Design review of the part built by this model. Coordinates are the model's own, in mm. A direction names the side the tool comes from. Give positions to 0.01 mm unless a question says otherwise; leave off trailing zeros. Order: outer loops, then holes, each group sorted by start corner. A loop starts at its lowest first (then second) coordinate and runs counter-clockwise, first axis right, second up. Notation, with made-up numbers: M -9.75,21 L 43.25,21 A21 cw 43.25,32 Z; hole C 57,86.5 d4. An arc over 180 degrees is marked long. Put each result on its own line as item: value. Start each with the question number.
from build123d import *

# Parameters (mm, degrees)
F0_R     = 1.75
F0_R_2   = 14
F1_DEPTH = 1
F2_W     = 21
F2_H     = 24
F3_DEPTH = 1.001
F4_R     = 2


with BuildPart() as f1:
    # F0 (on Top) → F1 (new body)
    with BuildSketch(Plane.XY):
        Polygon((15.3431457505, 21), (-15.3431457505, 21), (-21, 15.3431457505), (-21, -15.3431457505), (-15.3431457505, -21), (15.3431457505, -21), (21, -15.3431457505), (21, 15.3431457505), align=None)
        with Locations((-15.5, -15.5)):
            Circle(F0_R, mode=Mode.SUBTRACT)
        with Locations((15.5, -15.5)):
            Circle(F0_R, mode=Mode.SUBTRACT)
        with Locations((-15.5, 15.5)):
            Circle(F0_R, mode=Mode.SUBTRACT)
        Circle(F0_R_2, mode=Mode.SUBTRACT)
        with Locations((15.5, 15.5)):
            Circle(F0_R, mode=Mode.SUBTRACT)
    extrude(amount=F1_DEPTH)

    # F2 (on face) → F3 (cut, through all)
    with BuildSketch(Plane.XY.offset(1)):
        with Locations((10.5, 0)):
            Rectangle(F2_W, F2_H)
    extrude(amount=-F3_DEPTH, mode=Mode.SUBTRACT)

    # F4
    f4_edges = [f1.edges().sort_by_distance(p)[0] for p in [
        (7.211103, 12, 0.5),
        (21, 12, 0.5),
        (21, -12, 0.5),
        (7.211103, -12, 0.5),
    ]]
    fillet(f4_edges, radius=F4_R)


solid = f1.part
1. Consider section C-C on x = -9.5. Give the boundary of the cut face in (y, z).
2. To check wall thickness, follow probe 1 along Y at (x, z) = (13, 0.25); probe 2 along Y at (x, z) = (-15.5, 0.3); probe 3 along Y at (x, z) = (0, 0.5). State the ranges of each line that lie inside material, in increasing order.
3. Machinability: for faces 1 (the flat face through (-21, 0.2, 0.5)), 2 (the cylindrical face through (20.4, -12.57, 0.49)), 3 (the cylindrical face through (7.239, -12.065, 0.493)), which of the approach directions +Z, -Z, +X, -X, +Y, -Y give a long, thin tool a straight path to every point of the face, cutting with its end or side? Answer none if there is none.
4. The part is to be moulded in two halves that separate along X. For faces 4 (the cylindrical face through (7.253, 12.062, 0.493)), 5 (the flat face through (-18.211, -18.132, 0.493)), 6 (the flat face through (18.211, 18.132, 0.493)), 7 (the cylindrical face through (-14.6, 17, 0.5)), say which applies: +X half, -X half, draft (parallel to the pull), parting line (faces both ways), or undercut.
5. Consider section B-B on z = 0.65. Give the boundary of the cut face in (x, y), then the cut area to 3 significant figures.
6. Consider section A-A on x = 0. Give the boundary of the cut face in (y, z).
7. Insertion check: pin 1 (22.5 mm diameter, centred on x = 0, y = 0, fed in from +Z). The pin has a flat end and moves straight along its axis. Give the tip position at first contact, or say it passes through.
8. Consider section D-D on y = 0. Give the boundary of the cut face in (x, z), then the cut area to 3 significant figures.
Returned:
1. outline: M -21,0 L -10.28,0 L -10.28,1 L -21,1 Z; M 10.28,0 L 21,0 L 21,1 L 10.28,1 Z
2. probe 1: y = -21 to -12, 12 to 21
2. probe 2: y = -20.84 to -17.25, -13.75 to 13.75, 17.25 to 20.84
2. probe 3: y = -21 to -14, 14 to 21
3. face 1: +Z, -Z, -X, +Y, -Y
3. face 2: +Z, -Z, +X
3. face 3: +Z, -Z
4. face 4: undercut
4. face 5: -X half
4. face 6: +X half
4. face 7: undercut
5. outline: M -21,-15.34 L -15.34,-21 L 15.34,-21 L 21,-15.34 L 21,-14 A2 ccw 19,-12 L 7.75,-12 A2 ccw 6.78,-12.25 A14 cw long 6.78,12.25 A2 ccw 7.75,12 L 19,12 A2 ccw 21,14 L 21,15.34 L 15.34,21 L -15.34,21 L -21,15.34 Z; hole C -15.5,-15.5 d3.5; hole C -15.5,15.5 d3.5; hole C 15.5,-15.5 d3.5; hole C 15.5,15.5 d3.5
5. area: 828 mm2
6. outline: M -21,0 L -14,0 L -14,1 L -21,1 Z; M 14,0 L 21,0 L 21,1 L 14,1 Z
7. pin 1: passes through
8. outline: M -21,0 L -14,0 L -14,1 L -21,1 Z
8. area: 7.00 mm2
